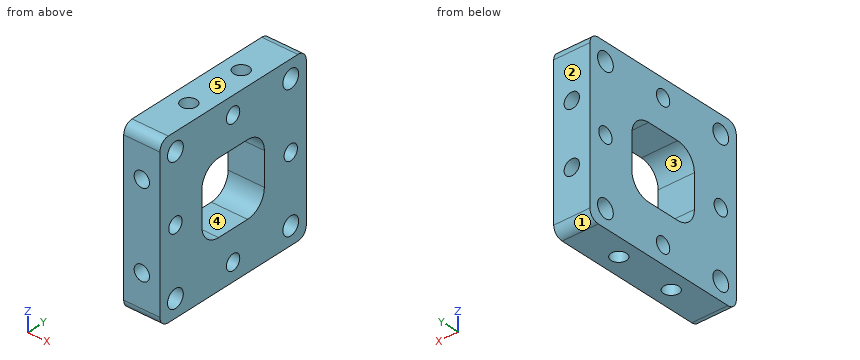
from build123d import *

# Parameters (mm, degrees)
SKETCH1_W                       = 44.323
SKETCH1_H                       = 44.323
SKETCH1_R                       = 2.38125
BOSS_EXTRUDE1_DEPTH             = 4.7625
FILLET1_R                       = 2.54
F_10_32_TAPPED_HOLE1_D          = 4.0386
F_10_32_TAPPED_HOLE1_DEPTH      = 12.0396
F_10_32_TAPPED_HOLE1_TIP        = 1.213317848
F_10_32_TAPPED_HOLE2_AT_2_COUNT = 2
F_10_32_TAPPED_HOLE2_AT_2_PITCH = 15.875
CIRPATTERN1_COUNT               = 4
F_10_32_TAPPED_HOLE3_D          = 4.0386
F_10_32_TAPPED_HOLE3_DEPTH      = 9.525
F_10_32_TAPPED_HOLE3_TIP        = 1.213317848
SKETCH19_W                      = 18.923
SKETCH19_H                      = 18.923
CUT_EXTRUDE1_DEPTH              = 33.756522854
FILLET2_R                       = 5.08


with BuildPart() as part:
    # Sketch1 → Boss-Extrude1 (new, symmetric)
    with BuildSketch(Plane(origin=(0, 0, 0), x_dir=(0, 0, -1), z_dir=(1, 0, 0))):
        Rectangle(SKETCH1_W, SKETCH1_H)
        with Locations(Location((-17.4625, 17.4625, 0), (0, 0, 180))):
            Circle(SKETCH1_R, mode=Mode.SUBTRACT)
        with Locations(Location((17.4625, 17.4625, 0), (0, 0, 180))):
            Circle(SKETCH1_R, mode=Mode.SUBTRACT)
        with Locations(Location((-17.4625, -17.4625, 0), (0, 0, 180))):
            Circle(SKETCH1_R, mode=Mode.SUBTRACT)
        with Locations(Location((17.4625, -17.4625, 0), (0, 0, 180))):
            Circle(SKETCH1_R, mode=Mode.SUBTRACT)
    extrude(amount=BOSS_EXTRUDE1_DEPTH, both=True)

    # Fillet1
    fillet1_edges = [part.edges().sort_by_distance(p)[0] for p in [
        (0, -22.1615, -22.1615),
        (0, -22.1615, 22.1615),
        (0, 22.1615, 22.1615),
        (0, 22.1615, -22.1615),
    ]]
    fillet(fillet1_edges, radius=FILLET1_R)

    # 10-32 Tapped Hole1
    with Locations(Plane.ZY.offset(4.7625)):
        with Locations((0, -17.4625), (0, 17.4625), (-17.4625, 0), (17.4625, 0)):
            Hole(F_10_32_TAPPED_HOLE1_D / 2, depth=F_10_32_TAPPED_HOLE1_DEPTH)
            with Locations((0, 0, -(F_10_32_TAPPED_HOLE1_DEPTH + F_10_32_TAPPED_HOLE1_TIP / 2))):  # 118° drill point
                Cone(0, F_10_32_TAPPED_HOLE1_D / 2, F_10_32_TAPPED_HOLE1_TIP, mode=Mode.SUBTRACT)

    # Sketch15 → 10-32 Tapped Hole2 (revolve, cut)
    with BuildSketch(Plane(origin=(0, 22.1615, -7.9375), x_dir=(0, 0, 1), z_dir=(1, 0, 0))):
        Polygon((0, 0), (0, 10.738317848), (2.0193, 9.525), (2.0193, 0), align=None)
    f_10_32_tapped_hole2 = revolve(axis=Axis((0, 28.5115, -7.9375), (0, -1, 0)), mode=Mode.SUBTRACT)

    # 10-32 Tapped Hole2 at 2: 10-32 Tapped Hole2 ×2
    with Locations(*[(0, 0, i * F_10_32_TAPPED_HOLE2_AT_2_PITCH) for i in range(1, F_10_32_TAPPED_HOLE2_AT_2_COUNT)]):
        add(f_10_32_tapped_hole2, mode=Mode.SUBTRACT)

    # CirPattern1: 10-32 Tapped Hole2 ×4 about axis, 1 skipped
    cirpattern1_axis = Axis((0, 0, 0), (1, 0, 0))
    add([f_10_32_tapped_hole2.rotate(cirpattern1_axis, i * 360 / CIRPATTERN1_COUNT) for i in range(1, CIRPATTERN1_COUNT) if i not in (2,)], mode=Mode.SUBTRACT)

    # CirPattern1 copy 1 sketch → CirPattern1 copy 1 (revolve, cut)
    with BuildSketch(Plane(origin=(0, -7.9375, 22.1615), x_dir=(0, -1, 0), z_dir=(1, 0, 0))):
        Polygon((0, 0), (0, 10.738317848), (2.0193, 9.525), (2.0193, 0), align=None)
    revolve(axis=Axis((0, -7.9375, 28.5115), (0, 0, -1)), mode=Mode.SUBTRACT)

    # CirPattern1 copy 2 sketch → CirPattern1 copy 2 (revolve, cut)
    with BuildSketch(Plane(origin=(0, 7.9375, -22.1615), x_dir=(0, 1, 0), z_dir=(1, 0, 0))):
        Polygon((0, 0), (0, 10.738317848), (2.0193, 9.525), (2.0193, 0), align=None)
    revolve(axis=Axis((0, 7.9375, -28.5115), (0, 0, 1)), mode=Mode.SUBTRACT)

    # 10-32 Tapped Hole3
    with Locations(Plane(origin=(0, -22.1615, 0), x_dir=(-1, 0, 0), z_dir=(0, -1, 0))):
        with Locations((0, -11.1125), (0, 11.1125)):
            Hole(F_10_32_TAPPED_HOLE3_D / 2, depth=F_10_32_TAPPED_HOLE3_DEPTH)
            with Locations((0, 0, -(F_10_32_TAPPED_HOLE3_DEPTH + F_10_32_TAPPED_HOLE3_TIP / 2))):  # 118° drill point
                Cone(0, F_10_32_TAPPED_HOLE3_D / 2, F_10_32_TAPPED_HOLE3_TIP, mode=Mode.SUBTRACT)

    # Sketch19 → Cut-Extrude1 (cut, through all)
    with BuildSketch(Plane(origin=(4.7625, 0, 0), x_dir=(0, 0, -1), z_dir=(1, 0, 0))):
        Rectangle(SKETCH19_W, SKETCH19_H)
    extrude(amount=-CUT_EXTRUDE1_DEPTH, mode=Mode.SUBTRACT)

    # Fillet2
    fillet2_edges = [part.edges().sort_by_distance(p)[0] for p in [
        (0, -9.4615, 9.4615),
        (0, 9.4615, 9.4615),
        (0, 9.4615, -9.4615),
        (0, -9.4615, -9.4615),
    ]]
    fillet(fillet2_edges, radius=FILLET2_R)


solid = part.part
Read the model definition and answer for the solid it produces. Units are mm, in the model's axes. Face numbers are marked on the shaded views. A direction names the side the tool comes from. Coordinates: 2 decimals unless noted, no trailing zeros. Write each loop counter-clockwise with the first axis right and the second up, starting at its lowest first coordinate (ties: lowest second). Pieces come first, ordered by that corner, then holes. Notation, with made-up numbers: (37.25, 33) - (45.25, 33) arc R29 ccw to (45.25, 59) - close; hole circle Ø7 at (44, 85). An arc over 180 degrees is marked (long way). One line per question, with ' | ' between items.
Q1. Find section C-C, the plane y = 18. Write down the section's boundary in (x, z), plus the area to 3 significant figures.
Result set:
outline: (-4.76, -22.16) - (4.76, -22.16) - (4.76, -19.78) - (-4.76, -19.78) - close; (-4.76, -15.14) - (4.76, -15.14) - (4.76, -1.95) - (-4.76, -1.95) - close; (-4.76, 1.95) - (4.76, 1.95) - (4.76, 15.14) - (-4.76, 15.14) - close; (-4.76, 19.78) - (4.76, 19.78) - (4.76, 22.16) - (-4.76, 22.16) - close; hole circle Ø4.04 at (0, -7.94); hole circle Ø4.04 at (0, 7.94) | area: 271 mm^2
Q2. For the marked faces 4 and 5, determine the directions among +Z, -Z, +X, -X, +Y, -Y from which every point of the face is accessible in a straight line to the end or side of a thin tool.
Result set:
face 4: +X, -X | face 5: +Z, +X, -X, +Y, -Y
Q3. Find section A-A, the plane z = 0. Write down the section's boundary in (x, y).
Result set:
outline: (-4.76, -22.16) - (4.76, -22.16) - (4.76, -19.48) - (-4.76, -19.48) - close; (-4.76, -15.44) - (4.76, -15.44) - (4.76, -9.46) - (-4.76, -9.46) - close; (-4.76, 9.46) - (4.76, 9.46) - (4.76, 15.44) - (-4.76, 15.44) - close; (-4.76, 19.48) - (4.76, 19.48) - (4.76, 22.16) - (-4.76, 22.16) - close
Q4. Find section D-D, the plane x = -3.5. State how many separate pieces and enclosed holes the cut face has, plus the area to 3 significant figures.
Result set:
separate pieces: 1 | enclosed holes: 9 | area: 1,500 mm^2
Q5. Each of these flat-tipped pins is pushed along its axis until it touches: P1, Ø2.5, axis at x = 0, y = -7.94, coming from the -Z side; P2, Ø3, axis at x = 0, y = 7.94, coming from the +Z side. Where does it stop, or does it pass through?
Result set:
P1: z = -12.18 | P2: z = 12.33
Q6. Consider L1, parallel to Y at x = 0, z = -15; L2, parallel to Z at x = -2.5, y = 17.5; L3, parallel to Z at x = 1.25, y = 13. Determine where each line is inside the solid, lowest interval first. Write a range as [from, to].
Result set:
L1: [-22.16, -9.96], [-5.92, 5.92], [9.96, 22.16] | L2: [-22.16, -19.84], [-15.08, -2.02], [2.02, 15.08], [19.84, 22.16] | L3: [-22.16, -9.52], [-6.35, 6.35], [9.52, 22.16]
Q7. Determine the mould class of the marked faces 1, 2 and 3 for opening direction Z: +Z half, -Z half, draft (parallel to the pull), parting line (faces both ways), or undercut.
Result set:
face 1: -Z half | face 2: draft | face 3: undercut
